Verification items for this drawing (mm, ordinates from the low corner). Round coordinates to 2 decimals unless told otherwise and drop trailing zeros. Order: outer loops, then holes, each group sorted by start corner. A loop starts at its lowest first (then second) coordinate and runs counter-clockwise, first axis right, second up. Notation, with made-up numbers: (36, 44.25) - (54, 44.25) arc R30 cw to (54, 74.25) - close; hole circle Ø8 at (36.25, 20.5). An arc over 180 degrees is marked (long way). Return JSON: item names as keys, results as strings. Group by question number.
Q1. Sectioned sample at B-B, the plane x = 0.95. Record the cut outline in (y, z).
Q2. Sectioned sample at D-D, the plane y = 1.75. Record the cut outline in (x, z).
Q3. Sectioned sample at C-C, the plane z = 0.9. Record the cut outline in (x, y), then the cut area to 3 significant figures.
Q4. Material ranges on line 1 along X through (y, z) = (2.25, 1.25); line 2 along Y through (x, z) = (0.8, 0.6); line 3 along Z through (x, y) = (2.2, 1.75), recorded low to high.
Q5. Sectioned sample at A-A, the plane y = 5. Record the cut outline in (x, z).
Q6. Gauge pin test, flat ends, axial feed: pin 1 Ø1 at (x, y) = (2.5, 5) entering from -Z; pin 2 Ø2 at (x, y) = (3.5, 1) entering from -Z. Record the tip position at first contact, or that the pin passes through.
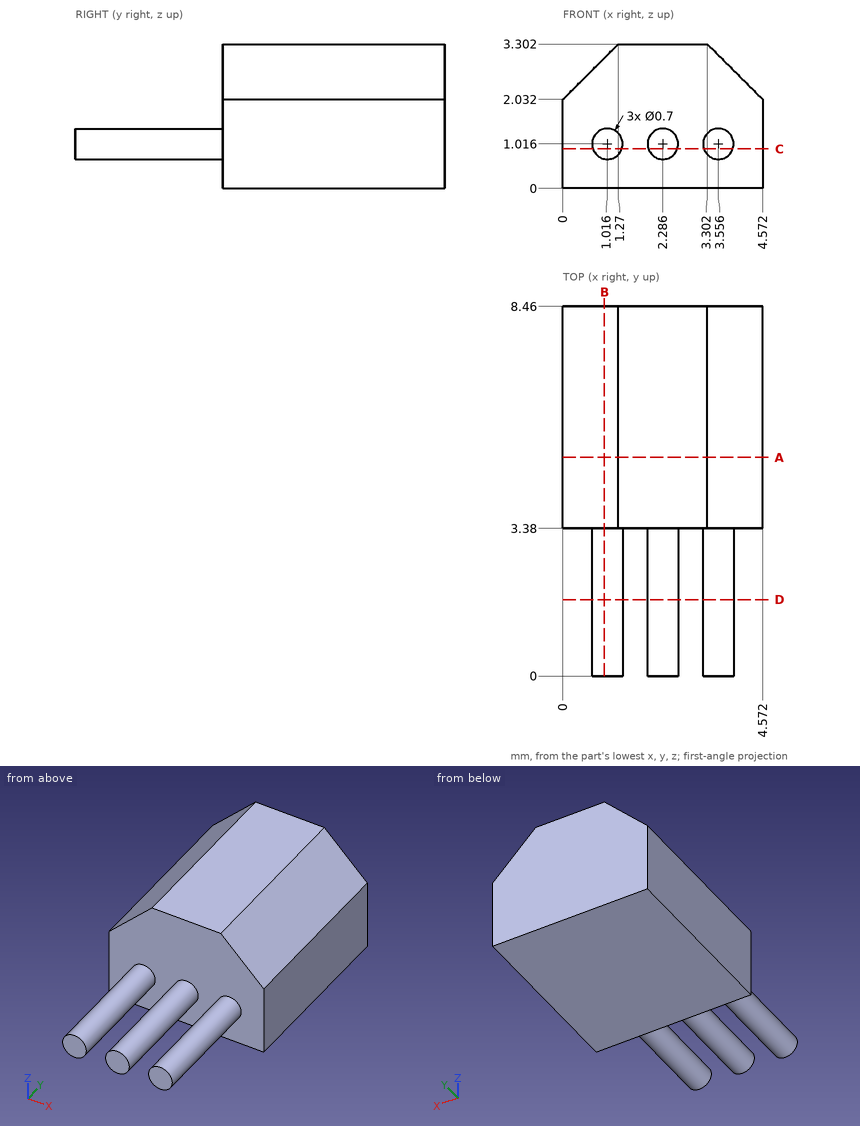
Reply:
{
 "1": {"outline": "(0, 0.67) - (3.38, 0.67) - (3.38, 0) - (8.46, 0) - (8.46, 2.98) - (3.38, 2.98) - (3.38, 1.36) - (0, 1.36) - close"},
 "2": {"outline": "circle Ø0.7 at (1.02, 1.02); circle Ø0.7 at (2.29, 1.02); circle Ø0.7 at (3.56, 1.02)"},
 "3": {"outline": "(0, 3.38) - (0.69, 3.38) - (0.69, 0) - (1.35, 0) - (1.35, 3.38) - (1.96, 3.38) - (1.96, 0) - (2.62, 0) - (2.62, 3.38) - (3.23, 3.38) - (3.23, 0) - (3.89, 0) - (3.89, 3.38) - (4.57, 3.38) - (4.57, 8.46) - (0, 8.46) - close", "area": "29.9 mm^2"},
 "4": {"line 1": "0.76 to 1.28, 2.03 to 2.55, 3.3 to 3.82", "line 2": "3.38 to 8.46", "line 3": "0.68 to 1.36"},
 "5": {"outline": "(0, 0) - (4.57, 0) - (4.57, 2.03) - (3.3, 3.3) - (1.27, 3.3) - (0, 2.03) - close"},
 "6": {"pin 1": "z = 0", "pin 2": "z = 0.67"}
}
